from build123d import *

# Parameters (mm, degrees)
F0_W           = 19.05
F0_H           = 82.55
F0_R           = 3.571875
F1_DEPTH       = 6.35
F2_D           = 6.7564
F2_CSINK_D     = 13.4874
F2_CSINK_ANGLE = 82


with BuildPart() as f1:
    # F0 (on Top) → F1 (new body)
    with BuildSketch(Plane.XY):
        Rectangle(F0_W, F0_H)
        with Locations((-3.175, -19.05)):
            Circle(F0_R, mode=Mode.SUBTRACT)
        with Locations((-3.175, 19.05)):
            Circle(F0_R, mode=Mode.SUBTRACT)
        with Locations((-3.175, 19.05)):
            Circle(F0_R)
        with Locations((-3.175, -19.05)):
            Circle(F0_R)
    extrude(amount=-F1_DEPTH)

    # F2 (through all)
    with Locations(Plane.XY):
        with Locations((-3.175, 19.05), (-3.175, -19.05)):
            CounterSinkHole(F2_D / 2, F2_CSINK_D / 2, counter_sink_angle=F2_CSINK_ANGLE)


solid = f1.part
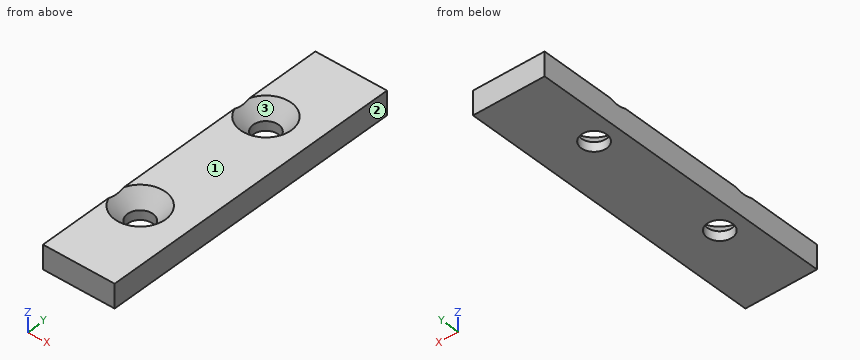
Geometry check sheet. Reference: the model listing, model coordinates, mm. Face numbers are marked on the shaded views. Round coordinates to 2 decimals unless told otherwise and drop trailing zeros. Write each loop counter-clockwise with the first axis right and the second up, starting at its lowest first coordinate (ties: lowest second). Pieces come first, ordered by that corner, then holes.
Item 1: Section check C-C (x = -3.75). Give the number of separate pieces and of enclosed holes in the cut face, plus the area to 3 significant figures.
Determined:
separate pieces: 3
enclosed holes: 0
area: 413 mm2
Item 2: Material ranges on line 1 along Y through (x, z) = (-3, -5) (3 decimals); line 2 along X through (y, z) = (-19.05, -4.45) (3 decimals); line 3 along Y through (x, z) = (-4.25, -2) (3 decimals), recorded low to high.
Determined:
line 1: y = -41.275 to -22.424, -15.676 to 15.676, 22.424 to 41.275
line 2: x = -9.525 to -6.553, 0.203 to 9.525
line 3: y = -41.275 to -23.938, -14.162 to 14.162, 23.938 to 41.275
Item 3: Section check A-A (y = 19.05). Record the boundary of the cut face in (x, z) (3 decimals).
Determined:
outline: (-9.525, -6.35) - (-6.553, -6.35) - (-6.553, -3.872) - (-9.525, -0.453) - close; (0.203, -6.35) - (9.525, -6.35) - (9.525, 0) - (3.569, 0) - (0.203, -3.872) - close
Item 4: Section check B-B (z = -2.25). Record the boundary of the cut face in (x, y) (3 decimals).
Determined:
outline: (-9.525, -41.275) - (9.525, -41.275) - (9.525, 41.275) - (-9.525, 41.275) - close; hole circle Ø9.576 at (-3.175, -19.05); hole circle Ø9.576 at (-3.175, 19.05)
Item 5: Mould release check, pull along X, two halves, no side actions. Record for the marked faces 1, 2 and 3: +X half, -X half, draft (parallel to the pull), parting line (faces both ways), or undercut.
Determined:
face 1: draft
face 2: +X half
face 3: undercut
Item 6: Go/stop test with a flat-tipped pin: pin 1 Ø1.5 at (x, y) = (-1, -3) entering from +Z. Record where the tip stops, or that it passes through.
Determined:
pin 1: stops at z = 0
